Geometry: final body of the model. Coordinates: model frame, mm. Face numbers are marked on the shaded views. A direction names the side the tool comes from. Give positions to 0.01 mm unless a question says otherwise; leave off trailing zeros. Write each loop counter-clockwise with the first axis right and the second up, starting at its lowest first coordinate (ties: lowest second). Pieces come first, ordered by that corner, then holes. Notation, with made-up numbers: M 0.25,36.5 L 47.25,36.5 A29 ccw 47.25,60.5 Z; hole C -11.5,35.5 d10. An arc over 180 degrees is marked long. Use a Markdown table: item, result. Add a question column.
1) Section A-A on x = 0. Return the cut outline in (y, z), then the cut area to 3 significant figures.
2) Line query: line 1 (Y direction, x = 0, z = -0.05); line 2 (Y direction, x = 5, z = 6.5); line 3 (Y direction, x = 0, z = 4.4). Output: solid intervals per line, ascending.
3) Section D-D on y = 3. Return the cut outline in (x, z).
4) Draft query along X for the marked faces 5, 6, 7 and 8. Return one class per face: +X half, -X half, draft (parallel to the pull), parting line (faces both ways), or undercut.
5) Section C-C on z = 14.75. State how many separate pieces and enclosed holes the cut face has, then the cut area to 3 significant figures.
6) Pin query (flat end, axial travel): pin 1 (2.5 mm diameter, centred on y = 9, z = 7, fed in from +X); pin 2 (3 mm diameter, centred on x = 7.5, z = 12, fed in from -Y); pin 3 (2.5 mm diameter, centred on x = -14, y = -3, fed in from +Z); pin 4 (3.5 mm diameter, centred on x = 14.5, y = 3, fed in from +Z). Return the tip coordinate at first contact, or that it passes through.
7) Section B-B on z = 2.75. Return the cut outline in (x, y), then the cut area to 3 significant figures.
8) Set-up query: the marked faces 1, 2, 3 and 4. Return all of +Z, -Z, +X, -X, +Y, -Y with unobstructed straight access to the full face (end or side cutting, diameter ignored); none if empty.
```python
from build123d import *
from build123d.topology import SkipClean

# Parameters (mm, degrees)
ESQUISSE1_R                  = 15.3
BOSS_EXTRU_1_DEPTH           = 3.5
ESQUISSE7_R                  = 15.3
ESQUISSE7_R_2                = 11
ESQUISSE7_R_3                = 3.5
BOSS_EXTRU_10_DEPTH          = 0.2
ESQUISSE2_R                  = 4
BOSS_EXTRU_2_DEPTH           = 6
ENL_V_MAT_EXTRU_2_DEPTH      = 24.631123545
ENL_V_MAT_EXTRU_2_DEPTH_BACK = 24.631123545
ESQUISSE4_R                  = 15.3
ESQUISSE4_R_2                = 13
BOSS_EXTRU_3_DEPTH           = 4
BOSS_EXTRU_4_DEPTH           = 8
R_P_TITION_CIRCULAIRE1_COUNT = 12
BOSS_EXTRU_9_DEPTH           = 0.5
R_P_TITION_CIRCULAIRE4_COUNT = 6


with BuildPart() as part:
    # Esquisse1 → Boss.-Extru.1 (new body)
    with BuildSketch(Plane.XY):
        Circle(ESQUISSE1_R)
    extrude(amount=BOSS_EXTRU_1_DEPTH)

    # Esquisse7 → Boss.-Extru.10 (add, symmetric)
    # profile 1 of 2: a face of its own
    with SkipClean():  # the faces are left unmerged after this step: merging them gives an invalid solid
        with BuildSketch(Plane(origin=(0, 0, 0), x_dir=(-1, 0, 0), z_dir=(0, 0, -1))):
            Circle(ESQUISSE7_R)
            with Locations(Location((0, 0, 0), (0, 0, 180))):
                Circle(ESQUISSE7_R_2, mode=Mode.SUBTRACT)
        # profile 2 of 2: a face of its own
        with BuildSketch(Plane(origin=(0, 0, 0), x_dir=(-1, 0, 0), z_dir=(0, 0, -1))):
            with Locations(Location((0, 0, 0), (0, 0, 180))):
                Circle(ESQUISSE7_R_3)
        extrude(amount=BOSS_EXTRU_10_DEPTH, both=True)

    # Esquisse2 → Boss.-Extru.2 (add)
    with SkipClean():  # the faces are left unmerged after this step: merging them gives an invalid solid
        with BuildSketch(Plane.XY.offset(3.5)):
            Circle(ESQUISSE2_R)
        extrude(amount=BOSS_EXTRU_2_DEPTH)

    # Esquisse3 → Enl_v. mat.-Extru.2 (cut, two sides: drawn at the far end of the back side and taken through both)
    with SkipClean():  # the faces are left unmerged after this step: merging them gives an invalid solid
        with BuildSketch(Plane.XY.offset(-ENL_V_MAT_EXTRU_2_DEPTH_BACK)):
            with BuildLine():
                Line((1, 1.118033989), (1, -1.118033989))
                ThreePointArc((1, -1.118033989), (-0.37200097, -1.4531398), (-1.414213562, -0.5))
                Line((-1.414213562, -0.5), (-8.414213562, -0.5))
                Line((-8.414213562, -0.5), (-8.414213562, 0.5))
                Line((-8.414213562, 0.5), (-1.414213562, 0.5))
                ThreePointArc((-1.414213562, 0.5), (-0.37200097, 1.4531398), (1, 1.118033989))
            make_face()
        extrude(amount=ENL_V_MAT_EXTRU_2_DEPTH + ENL_V_MAT_EXTRU_2_DEPTH_BACK, mode=Mode.SUBTRACT)

    # Esquisse4 → Boss.-Extru.3 (add)
    with SkipClean():  # the faces are left unmerged after this step: merging them gives an invalid solid
        with BuildSketch(Plane.XY.offset(3.5)):
            with Locations(Location((0, 0, 0), (0, 0, 180))):
                Circle(ESQUISSE4_R)
            Circle(ESQUISSE4_R_2, mode=Mode.SUBTRACT)
        extrude(amount=BOSS_EXTRU_3_DEPTH)

    # Esquisse5 → Boss.-Extru.4 (add)
    with SkipClean():  # the faces are left unmerged after this step: merging them gives an invalid solid
        with BuildSketch(Plane.XY.offset(7.5)):
            with BuildLine():
                Line((-1.647692308, 15.211019363), (-1.4, 12.924395537))
                ThreePointArc((-1.4, 12.924395537), (0, 13), (1.4, 12.924395537))
                Line((1.4, 12.924395537), (1.647692308, 15.211019363))
                ThreePointArc((1.647692308, 15.211019363), (0, 15.3), (-1.647692308, 15.211019363))
            make_face()
        boss_extru_4 = extrude(amount=BOSS_EXTRU_4_DEPTH)

    # R_p_tition circulaire1: Boss.-Extru.4 ×12 about axis
    with SkipClean():  # the faces are left unmerged after this step: merging them gives an invalid solid
        r_p_tition_circulaire1_axis = Axis((0, 0, 0), (0, 0, 1))
        for i in range(1, R_P_TITION_CIRCULAIRE1_COUNT):
            add(boss_extru_4.rotate(r_p_tition_circulaire1_axis, i * 360 / R_P_TITION_CIRCULAIRE1_COUNT))

    # Esquisse6 → Boss.-Extru.9 (add, symmetric)
    with SkipClean():  # the faces are left unmerged after this step: merging them gives an invalid solid
        with BuildSketch(Plane(origin=(0, 0, 0), x_dir=(0, 0, 1), z_dir=(1, 0, 0))):
            Polygon((8.833333333, 3), (5.5, 13), (3.5, 13), (3.5, 3), align=None)
        boss_extru_9 = extrude(amount=BOSS_EXTRU_9_DEPTH, both=True)

    # R_p_tition circulaire4: Boss.-Extru.9 ×6 about axis
    with SkipClean():  # the faces are left unmerged after this step: merging them gives an invalid solid
        r_p_tition_circulaire4_axis = Axis((0, 0, 0), (0, 0, 1))
        for i in range(1, R_P_TITION_CIRCULAIRE4_COUNT):
            add(boss_extru_9.rotate(r_p_tition_circulaire4_axis, i * 360 / R_P_TITION_CIRCULAIRE4_COUNT))


solid = part.part
```
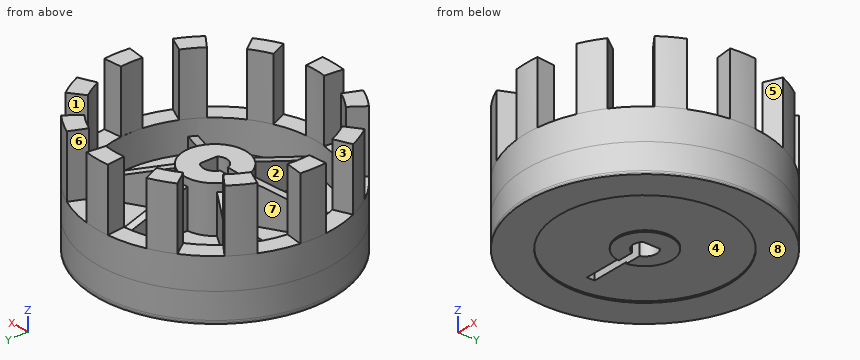
Found:
| question | item | result |
|---|---|---|
| 1 | outline | M -15.3,-0.2 L -11,-0.2 L -11,0 L -3.5,0 L -3.5,-0.2 L -1.5,-0.2 L -1.5,9.5 L -4,9.5 L -4,8.5 L -13,5.5 L -13,15.5 L -15.3,15.5 Z; M 1.5,-0.2 L 3.5,-0.2 L 3.5,0 L 11,0 L 11,-0.2 L 15.3,-0.2 L 15.3,15.5 L 13,15.5 L 13,5.5 L 4,8.5 L 4,9.5 L 1.5,9.5 Z |
| 1 | area | 247 mm² |
| 2 | line 1 | -15.3 to -11, -3.5 to -1.5, 1.5 to 3.5, 11 to 15.3 |
| 2 | line 2 | -14.46 to -12, -3.46 to -2.31, 2.31 to 3.46, 12 to 14.46 |
| 2 | line 3 | -15.3 to -1.5, 1.5 to 15.3 |
| 3 | outline | M -15,-0.2 L -10.58,-0.2 L -10.58,0 L -1.8,0 L -1.8,-0.2 L 1.8,-0.2 L 1.8,0 L 10.58,0 L 10.58,-0.2 L 15,-0.2 L 15,7.5 L 12.65,7.5 L 12.65,3.5 L 6.2,3.5 L 6.2,7.54 L 4.2,8.12 L 4.2,3.5 L 2.65,3.5 L 2.65,9.5 L -2.65,9.5 L -2.65,3.5 L -4.2,3.5 L -4.2,8.12 L -6.2,7.54 L -6.2,3.5 L -12.65,3.5 L -12.65,7.5 L -15,7.5 Z |
| 4 | face 5 | +X half |
| 4 | face 6 | undercut |
| 4 | face 7 | undercut |
| 4 | face 8 | draft |
| 5 | separate pieces | 12 |
| 5 | enclosed holes | 0 |
| 5 | area | 84.3 mm² |
| 6 | pin 1 | x = 13.19 |
| 6 | pin 2 | y = -14 |
| 6 | pin 3 | z = 7.5 |
| 6 | pin 4 | z = 15.5 |
| 7 | outline | C 0,0 d30.6; hole M -8.41,-0.5 L -1.41,-0.5 A1.5 ccw 1,-1.12 L 1,1.12 A1.5 ccw -1.41,0.5 L -8.41,0.5 Z |
| 7 | area | 722 mm² |
| 8 | face 1 | +Z, +Y |
| 8 | face 2 | +Z |
| 8 | face 3 | +Z, -X |
| 8 | face 4 | -Z |
